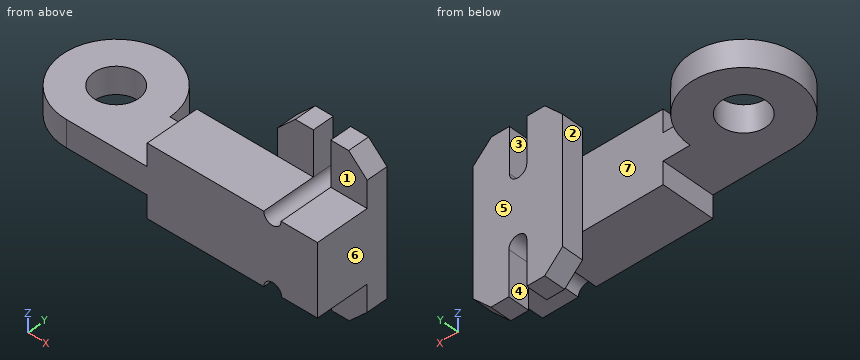
```python
from build123d import *

# Parameters (mm, degrees)
BOSS_EXTRUDE1_DEPTH = 12
SKETCH3_W           = 40
SKETCH3_H           = 30
BOSS_EXTRUDE2_DEPTH = 95
CUT_EXTRUDE1_START  = -95
SKETCH5_R           = 5
SKETCH5_R_2         = 4.855667385
CUT_EXTRUDE1_DEPTH  = 95
SKETCH7_R           = 12.5
BOSS_EXTRUDE3_DEPTH = 15


with BuildPart() as part:
    # Sketch1 → Boss-Extrude1 (new body)
    with BuildSketch(Plane(origin=(0, 0, 0), x_dir=(1, 0, 0), z_dir=(0, 1, 0))):
        with BuildLine():
            Line((-32.581308436, 24.430613363), (-42.581308436, 24.430613363))
            Line((-42.581308436, 24.430613363), (-52.581308436, 14.430613363))
            Line((-52.581308436, 14.430613363), (-52.581308436, -55.569386637))
            Line((-52.581308436, -55.569386637), (-42.581308436, -65.569386637))
            Line((-42.581308436, -65.569386637), (-32.581308436, -65.569386637))
            Line((-32.581308436, -65.569386637), (-32.581308436, -40.569386637))
            ThreePointArc((-32.581308436, -40.569386637), (-27.725641051, -35.713719251), (-22.869973665, -40.569386637))
            Line((-22.869973665, -40.569386637), (-22.869973665, -65.569386637))
            Line((-22.869973665, -65.569386637), (-12.869973665, -65.569386637))
            Line((-12.869973665, -65.569386637), (-2.581308436, -55.569386637))
            Line((-2.581308436, -55.569386637), (-2.581308436, 14.430613363))
            Line((-2.581308436, 14.430613363), (-12.581308436, 24.430613363))
            Line((-12.581308436, 24.430613363), (-22.581308436, 24.430613363))
            Line((-22.581308436, 24.430613363), (-22.581308436, -0.569386637))
            ThreePointArc((-22.581308436, -0.569386637), (-27.581308436, -5.569386637), (-32.581308436, -0.569386637))
            Line((-32.581308436, -0.569386637), (-32.581308436, 24.430613363))
        make_face()
    extrude(amount=BOSS_EXTRUDE1_DEPTH)

    # Sketch3 → Boss-Extrude2 (add)
    with BuildSketch(Plane(origin=(-2.581308436, 0, 0), x_dir=(0, 0, -1), z_dir=(1, 0, 0))):
        with Locations((-20.569386637, -15)):
            Rectangle(SKETCH3_W, SKETCH3_H)
    extrude(amount=-BOSS_EXTRUDE2_DEPTH)

    # Sketch5 → Cut-Extrude1 (cut)
    with BuildSketch(Plane(origin=(0, 12, 0), x_dir=(1, 0, 0), z_dir=(0, 1, 0)).offset(CUT_EXTRUDE1_START)):
        with Locations((-27.581308436, -0.569386637)):
            Circle(SKETCH5_R)
        with Locations((-27.725641051, -40.569386637)):
            Circle(SKETCH5_R_2)
    extrude(amount=CUT_EXTRUDE1_DEPTH, mode=Mode.SUBTRACT)

    # Sketch7 → Boss-Extrude3 (add)
    with BuildSketch(Plane(origin=(0, 0, 13.069386637), x_dir=(-1, 0, 0), z_dir=(0, 0, -1))):
        with BuildLine():
            Line((97.581308436, 0), (112.581308436, 0))
            ThreePointArc((112.581308436, 0), (163.794511872, 21.213203436), (142.581308436, -30))
            Line((142.581308436, -30), (97.581308436, -30))
            Line((97.581308436, -30), (97.581308436, 0))
        make_face()
        with Locations(Location((142.581308436, 0, 0), (0, 0, 90))):
            Circle(SKETCH7_R, mode=Mode.SUBTRACT)
    extrude(amount=-BOSS_EXTRUDE3_DEPTH)


solid = part.part
```
Source: CAD feature listing. Evaluate the final solid. Frame: model axes, mm. Face numbers are marked on the shaded views. A direction names the side the tool comes from. Coordinates: 2 decimals unless noted, no trailing zeros. Write each loop counter-clockwise with the first axis right and the second up, starting at its lowest first coordinate (ties: lowest second). Pieces come first, ordered by that corner, then holes. Notation, with made-up numbers: (-4, -11.5) -> (26, -11.5) arc R7 ccw to (26, -7.5) -> close; hole circle Ø9 at (78, 76.25). An arc over 180 degrees is marked (long way). Return JSON: item names as keys, results as strings. Group by question number.
1) Section query A-A, the plane z = 22. Return loops of the section in (x, y).
2) Section query D-D, the plane x = -57. Return loops of the section in (y, z).
3) Ray query, line 1 along X through (y, z) = (5.5, -5); line 2 along X through (y, z) = (-0.5, 17); line 3 along Z through (x, y) = (-61.5, -4). Return the intervals inside material, ascending.
4) Section query C-C, the plane y = 8.5. Return loops of the section in (x, z).
5) Mould query, pull axis X, two halves, no side actions, for the marked faces 5, 6 and 7. Classes: +X half, -X half, draft (parallel to the pull), parting line (faces both ways), or undercut.
6) Section query B-B, the plane z = -12.5. Return loops of the section in (x, y), plus the area to 3 significant figures.
7) Contact query for flat-ended pins moving along their axis: P1, Ø9.5, axis at y = 6, z = -15.5, coming from the -X side; P2, Ø1.5, axis at x = -104.5, y = -11, coming from the -Z side; P3, Ø16, axis at x = -10, y = -8.5, coming from the +Z side. Output: stop coordinate, or through.
8) Set-up query: the marked faces 1, 2, 3 and 4. Return all of +Z, -Z, +X, -X, +Y, -Y with unobstructed straight access to the full face (end or side cutting, diameter ignored); none if empty.
From the geometry:
{
 "1": {"outline": "(-142.58, -30) -> (-2.58, -30) -> (-2.58, 12) -> (-52.58, 12) -> (-52.58, 0) -> (-112.58, 0) arc R30 ccw (long way) to start; hole circle Ø25 at (-142.58, 0)"},
 "2": {"outline": "(-30, 0.57) -> (0, 0.57) -> (0, 40.57) -> (-30, 40.57) -> close"},
 "3": {"line 1": "-52.58 to -32.58, -22.58 to -2.58", "line 2": "-172.58 to -155.07, -130.09 to -2.58", "line 3": "0.57 to 40.57"},
 "4": {"outline": "(-171.35, 13.07) -> (-151.75, 13.07) -> (-151.75, 28.07) -> (-171.35, 28.07) -> close; (-133.42, 13.07) -> (-113.81, 13.07) -> (-113.81, 28.07) -> (-133.42, 28.07) -> close; (-52.58, -14.43) -> (-42.58, -24.43) -> (-32.58, -24.43) -> (-32.58, 0.57) arc R5 cw to (-22.58, 0.57) -> (-22.58, -24.43) -> (-12.58, -24.43) -> (-2.58, -14.43) -> (-2.58, 55.57) -> (-12.87, 65.57) -> (-22.87, 65.57) -> (-22.87, 40.57) arc R4.86 cw to (-32.58, 40.57) -> (-32.58, 65.57) -> (-42.58, 65.57) -> (-52.58, 55.57) -> close"},
 "5": {"face 5": "draft", "face 6": "+X half", "face 7": "undercut"},
 "6": {"outline": "(-52.58, 0) -> (-32.58, 0) -> (-32.58, 12) -> (-52.58, 12) -> close; (-22.58, 0) -> (-2.58, 0) -> (-2.58, 12) -> (-22.58, 12) -> close", "area": "480 mm²"},
 "7": {"P1": "x = -52.58", "P2": "z = 13.07", "P3": "z = 40.57"},
 "8": {"face 1": "+Z, +X, -X, -Y", "face 2": "+Z, -Z, +Y", "face 3": "+Z, +Y, -Y", "face 4": "-Z, +Y, -Y"}
}
